Could you check a few things on this model? Use its own coordinates, in mm. A direction names the side the tool comes from. Round coordinates to 2 decimals unless told otherwise and drop trailing zeros. Loops run counter-clockwise (first coordinate to the right, second up) from the corner with the lowest first, then second, coordinate; pieces in that order, holes last. Notation, with made-up numbers: (5, 17.5) -> (41, 17.5) arc R26 cw to (41, 53.5) -> close; hole circle Ø8 at (57, 18). An arc over 180 degrees is marked (long way). One line per item, written item: value.
Autodesk Inventor part; units mm, degrees
ref_plane "YZ Plane" through (0, 0, 0) normal (1, 0, 0) x (0, 1, 0)
ref_plane "XZ Plane" through (0, 0, 0) normal (0, 1, 0) x (-1, 0, 0)
ref_plane "XY Plane" through (0, 0, 0) normal (0, 0, 1) x (1, 0, 0)
sketch "Sketch1" plane through (0, 0, 0) normal (0, 1, 0) x (-1, 0, 0)
  line L0 (43.0361, 44.0554) -> (-25.9639, 44.0554)
  line L1 (-25.9639, 44.0554) -> (-25.9639, -34.9446)
  line L2 (-25.9639, -34.9446) -> (43.0361, -34.9446)
  line L3 (43.0361, -34.9446) -> (43.0361, 44.0554)
  point P0 (0, 0)
  dimension "d0" = 69
  dimension "d1" = 79
extrude "Extrusion1" add sketch "Sketch1" along normal blind 2.5
sketch "Sketch2" plane through (0, 2.5, 0) normal (0, 1, 0) x (1, 0, 0)
  circle A0 centre (23.9639, -42.0554) radius 1.2843
  line L0 (25.9639, -44.0554) -> (25.9639, 34.9446)
  line L1 (-43.0361, -44.0554) -> (25.9639, -44.0554)
  circle A1 centre (-41.0361, 2.9446) radius 1.3818
  circle A2 centre (23.9639, -14.0554) radius 1.5724
  line L2 (-43.0361, 34.9446) -> (-43.0361, -44.0554)
  line L3 (25.9639, 34.9446) -> (-43.0361, 34.9446)
  circle A3 centre (-8.5361, 32.9446) radius 1.5869
  circle A4 centre (-8.5361, -42.0554) radius 2.0414
  point P0 (0, 0)
  dimension "d4" = 2
  dimension "d5" = 2
  dimension "d26" = 2
  dimension "d27" = 2
  dimension "d28" = 32
  dimension "d29" = 30
  dimension "d37" = 2
  dimension "d38" = 2
  dimension "d39" = 34.5
  dimension "d40" = 34.5
hole "Hole1" at (23.9639, 2.5, 42.0554) direction (0, -1, 0) diameter 2.3 end through all counterbore diameter 3.3 counterbore depth 1.25
pattern_linear "Rectangular Pattern1" count 2 spacing 65 along (-1, 0, 0) count 2 spacing 75 along (0, 0, -1) of "Hole1"
sketch "Sketch3" plane through (0, 2.5, 0) normal (0, 1, 0) x (1, 0, 0)
  line L0 (5.4639, 28.1446) -> (20.4639, 28.1446)
  line L1 (21.9639, 26.6446) -> (21.9639, 12.1446)
  line L2 (20.4639, 10.6446) -> (5.4639, 10.6446)
  line L3 (3.9639, 12.1446) -> (3.9639, 26.6446)
  line L4 (-43.0361, -44.0554) -> (25.9639, -44.0554)
  line L5 (25.9639, -44.0554) -> (25.9639, 34.9446)
  arc A0 (5.4639, 28.1446) -> (3.9639, 26.6446) centre (5.4639, 26.6446) ccw
  arc A1 (21.9639, 26.6446) -> (20.4639, 28.1446) centre (20.4639, 26.6446) ccw
  arc A2 (20.4639, 10.6446) -> (21.9639, 12.1446) centre (20.4639, 12.1446) ccw
  arc A3 (3.9639, 12.1446) -> (5.4639, 10.6446) centre (5.4639, 12.1446) ccw
  point P0 (0, 0)
  point P1 (3.9639, 28.1446)
  point P2 (21.9639, 10.6446)
  point P3 (21.9639, 28.1446)
  point P4 (3.9639, 10.6446)
  dimension "d19" = 54.7
  dimension "d20" = 4
  dimension "d21" = 18
  dimension "d22" = 17.5
  dimension "d25" = 1.5
extrude "Extrusion2" cut sketch "Sketch3" against normal blind 2.5
hole "Hole2" at (-41.0361, 2.5, -2.9446) at (23.9639, 2.5, 14.0554) direction (0, -1, 0) diameter 2.3 end through all counterbore diameter 3.3 counterbore depth 1.25
hole "Hole3" at (-8.5361, 2.5, -32.9446) at (-8.5361, 2.5, 42.0554) direction (0, -1, 0) diameter 2.3 end through all counterbore diameter 3.3 counterbore depth 1.25
properties part number "Lid"
(1) We'd pull the mould along Z, two halves only. Please class faces 1 (the face through (-9, 1, 44.055)), 2 (the face through (13, 1, -28.145)), 3 (the face through (-8, 0, 5)): +Z half, -Z half, draft (parallel to the pull), parting line (faces both ways), or undercut.
Results below:
face 1: +Z half
face 2: undercut
face 3: draft
(2) Imagine slicing it at C-C on y = 0.65. Give the number of separate pieces and of enclosed holes in the cut face, then the cut area to 3 significant figures.
Results below:
separate pieces: 1
enclosed holes: 9
area: 5,100 mm²
(3) Imagine slicing it at A-A on z = -16.5. Write out the boundary of the cut face in (x, y).
Results below:
outline: (-43.04, 0) -> (3.96, 0) -> (3.96, 2.5) -> (-43.04, 2.5) -> close; (21.96, 0) -> (25.96, 0) -> (25.96, 2.5) -> (21.96, 2.5) -> close
(4) Imagine slicing it at B-B on x = 13. Write out the boundary of the cut face in (y, z), then the cut area to 3 significant figures.
Results below:
outline: (0, -34.94) -> (2.5, -34.94) -> (2.5, -28.14) -> (0, -28.14) -> close; (0, -10.64) -> (2.5, -10.64) -> (2.5, 44.06) -> (0, 44.06) -> close
area: 154 mm²
(5) Please list where these lines run through material, in increasing order: L1, parallel to Z at x = -10, y = 1.9; L2, parallel to X at y = 0.8, z = -21.5; L3, parallel to Z at x = -8.5, y = 1.4 (3 decimals).
Results below:
L1: z = -34.94 to -33.71, -32.18 to 41.29, 42.82 to 44.06
L2: x = -43.04 to 3.96, 21.96 to 25.96
L3: z = -34.945 to -34.594, -31.295 to 40.406, 43.705 to 44.055
(6) On a 3-axis mill with a long thin cutter (end or side, diameter ignored), from which of +Z, -Z, +X, -X, +Y, -Y can I reach the whole of each face in a straight line? I mean faces 4 (the face through (-8, 1, -34.945)), 5 (the face through (21.964, 1, -19)), 6 (the face through (-7.9, 1.87, -31.42)). Say none if no direction works.
Results below:
face 4: -Z, +X, -X, +Y, -Y
face 5: +Y, -Y
face 6: +Y
(7) For pin 1 Ø1.6 at (x, z) = (-8, 41.5) entering from +Y; pin 2 Ø1.6 at (x, z) = (-41, -3) entering from +Y, each with a flat end and sliding along its axis, tell me the tip position at first contact or that it passes through.
Results below:
pin 1: stops at y = 1.25
pin 2: passes through
